For this review, take the finished solid that the model builds, in its own axes (mm). A direction names the side the tool comes from. Give positions to 0.01 mm unless a question says otherwise; leave off trailing zeros. Loops run counter-clockwise (first coordinate to the right, second up) from the corner with the lowest first, then second, coordinate; pieces in that order, holes last.
```python
from build123d import *

# Parameters (mm, degrees)
BOSS_EXTRUDE1_DEPTH = 1
SKETCH1_3_W         = 1.9
SKETCH1_3_H         = 1.9
BOSS_EXTRUDE2_DEPTH = 3
SKETCH1_4_W         = 10.9395
SKETCH1_4_H         = 0.99
BOSS_EXTRUDE3_DEPTH = 50


with BuildPart() as part:
    # Sketch1 → Boss-Extrude1 (new body)
    with BuildSketch(Plane(origin=(0, 0, 0), x_dir=(1, 0, 0), z_dir=(0, 1, 0))):
        Polygon((-5.46975, -4.95), (0, -4.95), (5.46975, -4.95), (5.46975, 9.9), (-5.46975, 9.9), align=None)
    extrude(amount=BOSS_EXTRUDE1_DEPTH)

    # Sketch1<3> → Boss-Extrude2 (add)
    with BuildSketch(Plane(origin=(0, 0, 0), x_dir=(1, 0, 0), z_dir=(0, 1, 0))):
        with Locations((-4.51975, -0.95)):
            Rectangle(SKETCH1_3_W, SKETCH1_3_H)
        with Locations((4.51975, -0.95)):
            Rectangle(SKETCH1_3_W, SKETCH1_3_H)
    extrude(amount=-BOSS_EXTRUDE2_DEPTH)

    # Sketch1<4> → Boss-Extrude3 (add)
    with BuildSketch(Plane(origin=(0, 0, 0), x_dir=(1, 0, 0), z_dir=(0, 1, 0))):
        with Locations((0, 9.405)):
            Rectangle(SKETCH1_4_W, SKETCH1_4_H)
    extrude(amount=-BOSS_EXTRUDE3_DEPTH)


solid = part.part
```
Q1. For probe 1 along Z at (x, y) = (-4.5, -4); probe 2 along Y at (x, z) = (-5, 2); probe 3 along Y at (x, z) = (-3.75, 0.75), list the stretches that pass through material, from the lowest coordinate up.
Answers:
probe 1: z = -9.9 to -8.91
probe 2: y = 0 to 1
probe 3: y = -3 to 1
Q2. Consider section A-A on y = -1.5. Give the boundary of the cut face in (x, z), plus the area to 3 significant figures.
Answers:
outline: (-5.47, -9.9) - (5.47, -9.9) - (5.47, -8.91) - (-5.47, -8.91) - close; (-5.47, 0) - (-3.57, 0) - (-3.57, 1.9) - (-5.47, 1.9) - close; (3.57, 0) - (5.47, 0) - (5.47, 1.9) - (3.57, 1.9) - close
area: 18.1 mm2
Q3. Consider section C-C on x = 5. Give the boundary of the cut face in (y, z), plus the area to 4 significant figures.
Answers:
outline: (-50, -9.9) - (1, -9.9) - (1, 4.95) - (0, 4.95) - (0, 1.9) - (-3, 1.9) - (-3, 0) - (0, 0) - (0, -8.91) - (-50, -8.91) - close
area: 70.05 mm2
Q4. Mouldability with a two-part tool opening along X and no side actions: class faces 4 (the flat face through (3.57, -1, 1)), 5 (the flat face through (5.47, -16.8, -9.6)), 6 (the flat face through (-3.57, -1, 1)), 7 (the flat face through (-5, -3, 1)) as +X half, -X half, draft (parallel to the pull), parting line (faces both ways), or undercut.
Answers:
face 4: undercut
face 5: +X half
face 6: undercut
face 7: draft
Q5. Consider section D-D on x = 0.5. Give the boundary of the cut face in (y, z).
Answers:
outline: (-50, -9.9) - (1, -9.9) - (1, 4.95) - (0, 4.95) - (0, -8.91) - (-50, -8.91) - close
Q6. For pin 1 Ø6 at (x, z) = (-3.5, -4) entering from -Y; pin 2 Ø1 at (x, y) = (5, -1.5) entering from +Z; pin 3 Ø0.6 at (x, z) = (5, 1) entering from -Y, all flat-tipped, find the tip position at first contact; note any pin that passes through.
Answers:
pin 1: stops at y = 0
pin 2: stops at z = 1.9
pin 3: stops at y = -3
Q7. Consider section B-B on z = 1. Give the boundary of the cut face in (x, y).
Answers:
outline: (-5.47, -3) - (-3.57, -3) - (-3.57, 0) - (3.57, 0) - (3.57, -3) - (5.47, -3) - (5.47, 1) - (-5.47, 1) - close
Q8. Machinability: for faces 1 (the flat face through (5, -1, 0)), 2 (the flat face through (-5, -1, 1.9)), 3 (the flat face through (-5.47, -16.8, -9.6)), which of the approach directions +Z, -Z, +X, -X, +Y, -Y give a long, thin tool a straight path to every point of the face, cutting with its end or side? Answer none if there is none.
Answers:
face 1: +X, -X, -Y
face 2: +Z, +X, -X, -Y
face 3: +Z, -Z, -X, +Y, -Y
